Check sheet for the modelled part. Datum: model origin and axes. Units: mm. Coordinates: 2 decimals unless noted, no trailing zeros. Write each loop counter-clockwise with the first axis right and the second up, starting at its lowest first coordinate (ties: lowest second). Pieces come first, ordered by that corner, then holes. Notation, with made-up numbers: (-15.75, 70.25) - (30.25, 70.25) arc R16 ccw to (30.25, 93.25) - close; hole circle Ø5 at (-26, -38). An arc over 180 degrees is marked (long way). Answer as CSV lines item,"result". Start each with the question number.
from build123d import *

# Parameters (mm, degrees)
BOSS_EXTRU_1_DEPTH = 96
CONG_1_R           = 1


with BuildPart() as part:
    # Esquisse1 → Boss.-Extru.1 (new body)
    with BuildSketch(Plane.XY):
        with BuildLine():
            Line((0, 9), (58, 9))
            ThreePointArc((58, 9), (67, 0), (58, -9))
            Line((58, -9), (0, -9))
            ThreePointArc((0, -9), (-9, 0), (0, 9))
        make_face()
    extrude(amount=BOSS_EXTRU_1_DEPTH)

    # Congé1
    cong_1_edges = [part.edges().sort_by_distance(p)[0] for p in [
        (67, 0, 96),
        (29, 9, 96),
        (-9, 0, 96),
        (29, 9, 0),
        (67, 0, 0),
        (29, -9, 0),
        (-9, 0, 0),
        (29, -9, 96),
    ]]
    fillet(cong_1_edges, radius=CONG_1_R)


solid = part.part
(1) Go/stop test with a flat-tipped pin: P1, Ø6, axis at y = -3.5, z = 61, coming from the +X side. Record where the tip stops, or that it passes through.
(2) Material ranges on probe 1 along X at (y, z) = (-8, 47); probe 2 along X at (y, z) = (-6.5, 9.5); probe 3 along Y at (x, z) = (-1.5, 29.5), recorded low to high. Write a range as from..to.
(3) Release check for a two-part mould opening along X. For faces 1 (the face through (29, -9, 47)), 2 (the face through (-9, 0, 47)), 3 (the face through (67, 0, 47)) record: pulls with the +X half, pulls with the -X half, needs draft (parallel to the pull), parting line crosses it, or undercut.
(4) Cross-section at A-A on z = 66. Record the boundary of the cut face in (x, y).
Checked values:
1,P1,"x = 66.99"
2,probe 1,"-4.12..62.12"
2,probe 2,"-6.22..64.22"
2,probe 3,"-8.87..8.87"
3,face 1,"needs draft"
3,face 2,"pulls with the -X half"
3,face 3,"pulls with the +X half"
4,outline,"(0, -9) - (58, -9) arc R9 ccw to (58, 9) - (0, 9) arc R9 ccw to start"
